Check sheet for the modelled part. Datum: model origin and axes. Units: mm. A direction names the side the tool comes from. Coordinates: 2 decimals unless noted, no trailing zeros. Order: outer loops, then holes, each group sorted by start corner. A loop starts at its lowest first (then second) coordinate and runs counter-clockwise, first axis right, second up.
1. Set-up check for faces 5 (the cylindrical face through (-58, -115, 2)), 6 (the flat face through (56, 54.875, 2)), 7 (the flat face through (-56, -49.875, 2)): record each of +Z, -Z, +X, -X, +Y, -Y from which the full face is reachable in a straight line by a thin tool's end or side.
2. Thickness scan on line 1 (Y direction, x = -52.5, z = 0.8) (3 decimals); line 2 (Y direction, x = 51, z = 4.1); line 3 (X direction, y = -100, z = 0.3). Record the ranges inside material, lowest first.
3. Draft check along Y on faces 1 (the flat face through (-1, -116, 2)), 2 (the cylindrical face through (49.876, -52.43, 2.379)), 3 (the flat face through (60, -83, 2)), 4 (the cylindrical face through (-58, 59, 2)). Enter one of: released by +Y, released by -Y, zero draft, split by the parting line, or undercut.
4. Cross-section at A-A (x = 0). Enter the section's corners in (y, z), then the cut area to 3 significant figures.
5. Cross-section at B-B (y = -98.5). Enter the section's corners in (x, z), then the cut area to 3 significant figures.
6. Gauge pin test, flat ends, axial feed: pin 1 Ø2.5 at (x, z) = (-56.5, 2) entering from -Y; pin 2 Ø2.5 at (x, y) = (42.975, -85.525) entering from +Z; pin 3 Ø2.5 at (x, z) = (58, 2.5) entering from +Y; pin 4 Ø1.5 at (y, z) = (-53, 4) entering from +X. Record the tip position at first contact, or that the pin passes through.
```python
from build123d import *

# Parameters (mm, degrees)
F1_R     = 3.5
F1_R_2   = 1.4732
F2_DEPTH = 4.826
F3_R     = 5


with BuildPart() as f2:
    # F1 (on face) → F2 (new body)
    with BuildSketch(Plane.XY):
        with BuildLine():
            Line((60, 54.875), (60, 60))
            Line((60, 60), (-60, 60))
            Line((-60, 60), (-60, 54.875))
            Line((-60, 54.875), (-52.375, 54.875))
            ThreePointArc((-52.375, 54.875), (-50.607233, 54.142767), (-49.875, 52.375))
            ThreePointArc((-49.875, 52.375), (-50.607233, 50.607233), (-52.375, 49.875))
            Line((-52.375, 49.875), (-60, 49.875))
            Line((-60, 49.875), (-60, -49.875))
            Line((-60, -49.875), (-52.375, -49.875))
            ThreePointArc((-52.375, -49.875), (-50.607233, -50.607233), (-49.875, -52.375))
            ThreePointArc((-49.875, -52.375), (-50.607233, -54.142767), (-52.375, -54.875))
            Line((-52.375, -54.875), (-60, -54.875))
            Line((-60, -54.875), (-60, -60))
            Line((-60, -60), (-60, -116))
            Line((-60, -116), (60, -116))
            Line((60, -116), (60, -60))
            Line((60, -60), (60, -54.875))
            Line((60, -54.875), (52.375, -54.875))
            ThreePointArc((52.375, -54.875), (49.875, -52.375), (52.375, -49.875))
            Line((52.375, -49.875), (60, -49.875))
            Line((60, -49.875), (60, 49.875))
            Line((60, 49.875), (52.375, 49.875))
            ThreePointArc((52.375, 49.875), (49.875, 52.375), (52.375, 54.875))
            Line((52.375, 54.875), (60, 54.875))
        make_face()
        with Locations((0, -98.5)):
            Circle(F1_R, mode=Mode.SUBTRACT)
        with Locations((17.025, -111.475)):
            Circle(F1_R_2, mode=Mode.SUBTRACT)
        with Locations((17.025, -85.525)):
            Circle(F1_R_2, mode=Mode.SUBTRACT)
        with Locations((42.975, -111.475)):
            Circle(F1_R_2, mode=Mode.SUBTRACT)
        with Locations((42.975, -85.525)):
            Circle(F1_R_2, mode=Mode.SUBTRACT)
    extrude(amount=F2_DEPTH)

    # F3
    f3_edges = [f2.edges().sort_by_distance(p)[0] for p in [
        (-60, 60, 2.413),
        (60, 60, 2.413),
        (60, -116, 2.413),
        (-60, -116, 2.413),
    ]]
    fillet(f3_edges, radius=F3_R)


solid = f2.part
```
Data:
1. face 5: +Z, -Z, -X, -Y
1. face 6: +Z, -Z, +X
1. face 7: +Z, -Z, -X
2. line 1: y = -116 to -54.875, -49.875 to 49.875, 54.875 to 60
2. line 2: y = -116 to -54.46, -50.29 to 50.29, 54.46 to 60
2. line 3: x = -60 to -3.16, 3.16 to 60
3. face 1: released by -Y
3. face 2: undercut
3. face 3: zero draft
3. face 4: released by +Y
4. outline: (-116, 0) - (-102, 0) - (-102, 4.83) - (-116, 4.83) - close; (-95, 0) - (60, 0) - (60, 4.83) - (-95, 4.83) - close
4. area: 816 mm2
5. outline: (-60, 0) - (-3.5, 0) - (-3.5, 4.83) - (-60, 4.83) - close; (3.5, 0) - (60, 0) - (60, 4.83) - (3.5, 4.83) - close
5. area: 545 mm2
6. pin 1: stops at y = -115.99
6. pin 2: passes through
6. pin 3: stops at y = 59.68
6. pin 4: stops at x = 50.29
